Here's how the part is built. I have some questions about the finished solid (model axes, mm). Round coordinates to 2 decimals unless told otherwise and drop trailing zeros. Order: outer loops, then holes, each group sorted by start corner. A loop starts at its lowest first (then second) coordinate and runs counter-clockwise, first axis right, second up.
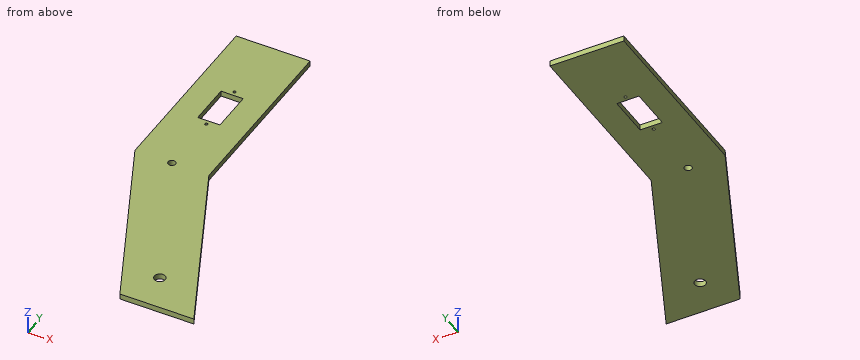
```python
from build123d import *

# Parameters (mm, degrees)
CROQUIS1_R              = 2.95
CROQUIS1_R_2            = 0.75
CROQUIS1_R_3            = 2
CROQUIS1_W              = 12
CROQUIS1_H              = 23
SALIENTE_EXTRUIR1_DEPTH = 3


with BuildPart() as part:
    # Croquis1 → Saliente-Extruir1 (new body)
    with BuildSketch(Plane.XY):
        Polygon((0, 0), (-40, 0), (-86.630765816, 100), (-86.630765816, 200), (-46.630765816, 200), (-46.630765816, 100), align=None)
        with Locations((-29.326153163, 20)):
            Circle(CROQUIS1_R, mode=Mode.SUBTRACT)
        with Locations((-66.630765816, 133.95806763)):
            Circle(CROQUIS1_R_2, mode=Mode.SUBTRACT)
        with Locations((-66.630765816, 161.95806763)):
            Circle(CROQUIS1_R_2, mode=Mode.SUBTRACT)
        with Locations((-66.630765816, 100)):
            Circle(CROQUIS1_R_3, mode=Mode.SUBTRACT)
        with Locations((-66.630765816, 147.95806763)):
            Rectangle(CROQUIS1_W, CROQUIS1_H, mode=Mode.SUBTRACT)
    extrude(amount=SALIENTE_EXTRUIR1_DEPTH)


solid = part.part
```
1) If we section it at B-B (z = 2.15): Write out the boundary of the cut face in (x, y).
2) I need wall thicknesses on line 1 (Y direction, x = -67, z = 0.4); line 2 (X direction, y = 111, z = 1.65); line 3 (X direction, y = 153, z = 1.05). Which ranges of each line are inside material? Lowest first, please.
3) If we section it at A-A (y = 155.5): Write out the boundary of the cut face in (x, z).
4) If we section it at C-C (y = 20): Write out the boundary of the cut face in (x, z), plus the area to 3 significant figures.
5) If we section it at D-D (x = -37): Write out the boundary of the cut face in (y, z).
6) I'm going to push flat-ended pins straight in: pin 1 (1 mm diameter, centred on y = 108.5, z = 0.5, fed in from +X); pin 2 (5 mm diameter, centred on x = -29.5, y = 26, fed in from -Z); pin 3 (0.9 mm diameter, centred on x = -66.63, y = 133.96, fed in from -Z); pin 4 (1 mm diameter, centred on x = -53, z = 1.5, fed in from -Y). Where does each tip first touch, or does it pass through?
Solutions:
1. outline: (-86.63, 100) - (-40, 0) - (0, 0) - (-46.63, 100) - (-46.63, 200) - (-86.63, 200) - close; hole (-72.63, 136.46) - (-60.63, 136.46) - (-60.63, 159.46) - (-72.63, 159.46) - close; hole circle Ø4 at (-66.63, 100); hole circle Ø1.5 at (-66.63, 133.96); hole circle Ø1.5 at (-66.63, 161.96); hole circle Ø5.9 at (-29.33, 20)
2. line 1: y = 57.9 to 98.03, 101.97 to 133.31, 134.61 to 136.46, 159.46 to 161.31, 162.61 to 200
2. line 2: x = -86.63 to -46.63
2. line 3: x = -86.63 to -72.63, -60.63 to -46.63
3. outline: (-86.63, 0) - (-72.63, 0) - (-72.63, 3) - (-86.63, 3) - close; (-60.63, 0) - (-46.63, 0) - (-46.63, 3) - (-60.63, 3) - close
4. outline: (-49.33, 0) - (-32.28, 0) - (-32.28, 3) - (-49.33, 3) - close; (-26.38, 0) - (-9.33, 0) - (-9.33, 3) - (-26.38, 3) - close
4. area: 102 mm2
5. outline: (0, 0) - (79.35, 0) - (79.35, 3) - (0, 3) - close
6. pin 1: stops at x = -46.63
6. pin 2: stops at z = 0
6. pin 3: passes through
6. pin 4: stops at y = 26.81
